The listing builds one solid part. Answer for the finished solid, in the listing's coordinates (mm). Give positions to 0.01 mm unless a question says otherwise; leave off trailing zeros. Write each loop counter-clockwise with the first axis right and the second up, starting at its lowest first coordinate (ties: lowest second). Pieces come first, ordered by that corner, then holes. Notation, with made-up numbers: (10, 73.25) -> (48, 73.25) arc R16 cw to (48, 91.25) -> close; hole circle Ø6 at (-1.5, 59). An arc over 180 degrees is marked (long way). One line per question, with ' | ' between items.
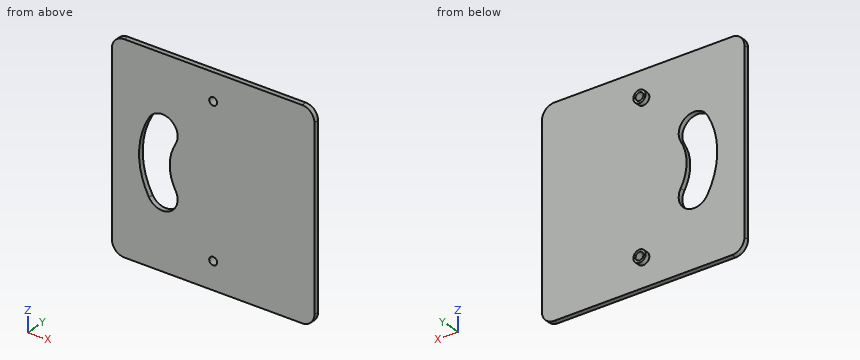
Autodesk Inventor part; units mm, degrees
ref_plane "YZ Plane" through (0, 0, 0) normal (1, 0, 0) x (0, 1, 0)
ref_plane "XZ Plane" through (0, 0, 0) normal (0, 1, 0) x (-1, 0, 0)
ref_plane "XY Plane" through (0, 0, 0) normal (0, 0, 1) x (1, 0, 0)
sketch "Sketch1" plane through (0, 0, 0) normal (0, 1, 0) x (-1, 0, 0)
  line L0 (32.8496, 31.7326) -> (-49.1504, 31.7326)
  line L1 (-49.1504, 31.7326) -> (-49.1504, -50.2674)
  line L2 (-49.1504, -50.2674) -> (32.8496, -50.2674)
  line L3 (32.8496, -50.2674) -> (32.8496, 31.7326)
  circle A0 centre (-8.1504, -9.2674) radius 30
  circle A1 centre (-8.1504, -39.2674) radius 2.5
  circle A2 centre (-8.1504, 20.7326) radius 2.5
  circle A3 centre (-8.1504, -39.2674) radius 1.6
  circle A4 centre (-8.1504, 20.7326) radius 1.6
  arc A5 (12.448, -21.16) -> (12.4481, 2.625) centre (-8.1504, -9.2674) ccw construction
  arc A6 (17.8304, -24.2675) -> (17.8305, 5.7325) centre (-8.1504, -9.2674) ccw
  arc A7 (7.0656, -18.0524) -> (7.0657, -0.4825) centre (-8.1504, -9.2674) ccw
  arc A8 (7.0656, -18.0524) -> (17.8304, -24.2675) centre (12.448, -21.16) ccw
  arc A9 (17.8305, 5.7325) -> (7.0657, -0.4825) centre (12.4481, 2.625) ccw
  line L4 (-8.1504, -9.2674) -> (12.448, -21.16) construction
  line L5 (-8.1504, -9.2674) -> (12.4481, 2.625) construction
  point P0 (0, 0)
  point P1 (17.8304, -24.2675)
  point P2 (17.8305, 5.7325)
  dimension "d0" = 82
  dimension "d1" = 82
  dimension "d2" = 60
  dimension "d3" = 5
  dimension "d4" = 5
  dimension "d5" = 3.2
  dimension "d6" = 3.2
  dimension "d7" = 60
extrude "Extrusion1" add sketch "Sketch1" along normal blind 2 contours L3 L2 L1 L0 | A9 A7 A8 A0 A1 A2
extrude "Extrusion2" add sketch "Sketch1" along normal blind 4 contours A2 A0 A4 | A0 A4 A2 | A1 A0 A3 | A0 A3 A1
sketch "Sketch2" plane through (0, 2, 0) normal (0, 1, 0) x (1, 0, 0)
  line L0 (49.1504, -31.7326) -> (49.1504, 50.2674)
  line L1 (49.1504, 50.2674) -> (-32.8496, 50.2674)
  line L2 (-32.8496, 50.2674) -> (-32.8496, -31.7326)
  line L3 (-32.8496, -31.7326) -> (49.1504, -31.7326)
  circle A0 centre (8.1504, -20.7326) radius 2.5
  circle A1 centre (8.1504, 39.2674) radius 2.5
  arc A2 (-7.0656, 18.0524) -> (-17.8304, 24.2675) centre (-12.448, 21.16) ccw
  arc A3 (-7.0656, 18.0524) -> (-7.0657, 0.4825) centre (8.1504, 9.2674) ccw
  arc A4 (-17.8305, -5.7325) -> (-7.0657, 0.4825) centre (-12.4481, -2.625) ccw
  arc A5 (-17.8304, 24.2675) -> (-17.8305, -5.7325) centre (8.1504, 9.2674) ccw
  circle A6 centre (-27.8496, 45.2674) radius 5
  circle A7 centre (-27.8496, -26.7326) radius 5
  circle A8 centre (44.1504, 45.2674) radius 5
  circle A9 centre (44.1504, -26.7326) radius 5
  point P0 (0, 0)
  point P1 (-27.8496, -31.7326)
  point P2 (-32.8496, -26.7326)
  point P3 (49.1504, -26.7326)
  point P4 (44.1504, -31.7326)
  point P5 (44.1504, 50.2674)
  point P6 (49.1504, 45.2674)
  point P7 (-32.8496, 45.2674)
  point P8 (-27.8496, 50.2674)
  dimension "d12" = 10
  dimension "d13" = 0
  dimension "d14" = 0
  dimension "d15" = 10
  dimension "d16" = 0
  dimension "d17" = 10
  dimension "d18" = 0
  dimension "d19" = 10
extrude "Extrusion3" cut sketch "Sketch2" along normal mid plane 4 contours L3 A9 L0 | A8 L1 L0 | L3 L2 A7 | A6 L2 L1
sketch "Sketch3" plane through (0, 2, 0) normal (0, 1, 0) x (1, 0, 0)
  line L0 (44.1504, 50.2674) -> (-27.8496, 50.2674)
  line L1 (-27.8496, -31.7326) -> (44.1504, -31.7326)
  point P0 (0, 0)
  dimension "d22" = 82
properties part number "controler_01"
Item 1: Consider line 1 (X direction, y = 1.5, z = -39.5); line 2 (Z direction, x = 9, y = 1.2); line 3 (Z direction, x = 6, y = 3.25). Determine where each line is inside the solid, lowest interval first. Write a range as [from, to].
Answers below:
line 1: [-32.85, 6.57], [9.73, 49.15] | line 2: [-50.27, -40.62], [-37.91, 19.38], [22.09, 31.73] | line 3: [-40.54, -37.99], [19.46, 22.01]
Item 2: Find section D-D (z = 15.5). Write down the section's boundary in (x, y), then the cut area to 3 significant figures.
Answers below:
outline: (-32.85, 0) -> (49.15, 0) -> (49.15, 2) -> (-32.85, 2) -> close | area: 164 mm²
Item 3: Find section B-B (x = -12.5). Write down the section's boundary in (y, z).
Answers below:
outline: (0, -50.27) -> (2, -50.27) -> (2, -27.37) -> (0, -27.37) -> close; (0, 8.84) -> (2, 8.84) -> (2, 31.73) -> (0, 31.73) -> close
Item 4: Flat-ended cylindrical pins translate along their axes: pin 1 (2 mm diameter, centred on x = -4.5, z = -24.5, fed in from -Y); pin 2 (1.5 mm diameter, centred on x = 35, z = 11, fed in from +Y); pin 3 (3 mm diameter, centred on x = 8.15, z = 20.73, fed in from +Y). Find the tip coordinate at first contact, or state that the pin passes through.
Answers below:
pin 1: y = 0 | pin 2: y = 2 | pin 3: through
Item 5: Find section A-A (z = -21.5). Write down the section's boundary in (x, y), then the cut area to 3 significant figures.
Answers below:
outline: (-32.85, 0) -> (-19.24, 0) -> (-19.24, 2) -> (-32.85, 2) -> close; (-6.24, 0) -> (49.15, 0) -> (49.15, 2) -> (-6.24, 2) -> close | area: 138 mm²
Item 6: Find section C-C (y = 0.95). Write down the section's boundary in (x, z) (1 decimal), then the cut area to 3 significant figures.
Answers below:
outline: (-32.8, -45.3) arc R5 ccw to (-27.8, -50.3) -> (44.2, -50.3) arc R5 ccw to (49.2, -45.3) -> (49.2, 26.7) arc R5 ccw to (44.2, 31.7) -> (-27.8, 31.7) arc R5 ccw to (-32.8, 26.7) -> close; hole (-17.8, -24.3) arc R6.2 ccw to (-7.1, -18.1) arc R17.6 cw to (-7.1, -0.5) arc R6.2 ccw to (-17.8, 5.7) arc R30 ccw to start; hole circle Ø3.2 at (8.2, -39.3); hole circle Ø3.2 at (8.2, 20.7) | area: 6,260 mm²
